Part model, mm, in its own coordinate system. Give positions to 0.01 mm unless a question says otherwise; leave off trailing zeros. Order: outer loops, then holes, each group sorted by start corner. A loop starts at its lowest first (then second) coordinate and runs counter-clockwise, first axis right, second up. Notation, with made-up numbers: (60, 21) - (89, 21) arc R20 cw to (89, 60) - close; hole circle Ø5 at (17, -21). An arc over 180 degrees is marked (long way). One line per item, written item: value.
```python
from build123d import *

# Parameters (mm, degrees)
SKETCH1_W           = 150
SKETCH1_H           = 75
BOSS_EXTRUDE1_DEPTH = 5
SKETCH2_W           = 7.5
SKETCH2_H           = 7.5
BOSS_EXTRUDE2_DEPTH = 2
SKETCH3_W           = 4
SKETCH3_H           = 7.5
BOSS_EXTRUDE3_DEPTH = 7
FILLET1_R           = 2
SKETCH6_R           = 2
CUT_EXTRUDE1_DEPTH  = 5


with BuildPart() as part:
    # Sketch1 → Boss-Extrude1 (new body)
    with BuildSketch(Plane.XY):
        Rectangle(SKETCH1_W, SKETCH1_H)
    extrude(amount=BOSS_EXTRUDE1_DEPTH)

    # Sketch2 → Boss-Extrude2 (add)
    with BuildSketch(Plane(origin=(0, 0, 0), x_dir=(-1, 0, 0), z_dir=(0, 0, -1))):
        Rectangle(SKETCH2_W, SKETCH2_H)
    extrude(amount=BOSS_EXTRUDE2_DEPTH)

    # Sketch3 → Boss-Extrude3 (add)
    with BuildSketch(Plane(origin=(0, 0, -2), x_dir=(-1, 0, 0), z_dir=(0, 0, -1))):
        Rectangle(SKETCH3_W, SKETCH3_H)
    extrude(amount=BOSS_EXTRUDE3_DEPTH)

    # Fillet1
    fillet1_edges = [part.edges().sort_by_distance(p)[0] for p in [
        (0, 3.75, -9),
        (0, -3.75, -9),
    ]]
    fillet(fillet1_edges, radius=FILLET1_R)

    # Sketch6 → Cut-Extrude1 (cut)
    with BuildSketch(Plane(origin=(2, 0, 0), x_dir=(0, 0, -1), z_dir=(1, 0, 0))):
        with Locations((6, 0)):
            Circle(SKETCH6_R)
    extrude(amount=-CUT_EXTRUDE1_DEPTH, mode=Mode.SUBTRACT)


solid = part.part
```
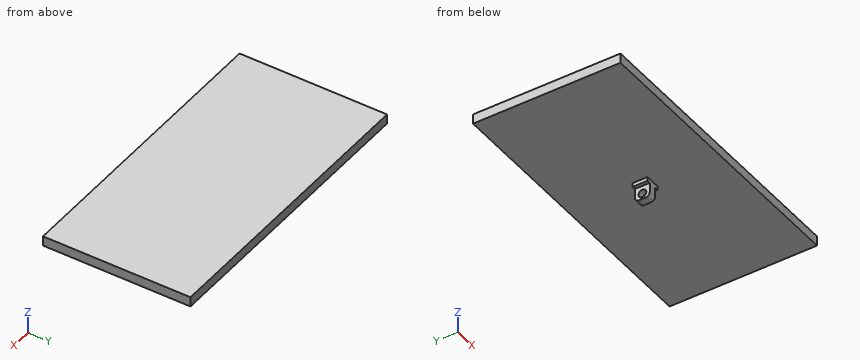
1) Slice it at A-A on y = 0. Write the cut outline in (x, z), then the cut area to 3 significant figures.
Answer:
outline: (-75, 0) - (-3.75, 0) - (-3.75, -2) - (-2, -2) - (-2, -4) - (2, -4) - (2, -2) - (3.75, -2) - (3.75, 0) - (75, 0) - (75, 5) - (-75, 5) - close; (-2, -9) - (2, -9) - (2, -8) - (-2, -8) - close
area: 777 mm2
2) Drop flat-ended pins along their axis: P1, Ø1.4, axis at x = 3, y = 0.5, coming from the -Z side; P2, Ø3.5, axis at y = -0.5, z = -4, coming from the -X side; P3, Ø7.5, axis at y = 0.5, z = -6, coming from the +X side. Give the stop position or say it passes through.
Answer:
P1: stops at z = -2
P2: stops at x = -2
P3: stops at x = 2
3) Slice it at B-B on y = -20.5. Write the cut outline in (x, z), then the cut area to 3 significant figures.
Answer:
outline: (-75, 0) - (75, 0) - (75, 5) - (-75, 5) - close
area: 750 mm2
4) Slice it at C-C on x = 52. Write the cut outline in (y, z), then the cut area to 3 significant figures.
Answer:
outline: (-37.5, 0) - (37.5, 0) - (37.5, 5) - (-37.5, 5) - close
area: 375 mm2
5) Wall check: line 1 along Y through (x, z) = (-0.15, -6); line 2 along X through (y, z) = (-1, -0.75); line 3 along Z through (x, y) = (9, -0.5). Give the ranges that are in metal, low to high. Write a range as [from, to].
Answer:
line 1: y = [-3.75, -2], [2, 3.75]
line 2: x = [-3.75, 3.75]
line 3: z = [0, 5]
